Input: part model. Units: mm. Frame: model coordinates. A direction names the side the tool comes from. Round coordinates to 2 decimals unless told otherwise and drop trailing zeros. Order: outer loops, then holes, each group sorted by start corner. A loop starts at its lowest first (then second) coordinate and runs counter-clockwise, first axis right, second up. Notation, with made-up numbers: (50.25, 31.25) -> (59.25, 31.25) arc R31 ccw to (59.25, 60.25) -> close; hole circle Ø3 at (24.5, 38). An arc over 180 degrees is marked (long way). Use a Markdown table: item, result.
from build123d import *

# Parameters (mm, degrees)
F1_R     = 11
F1_R_2   = 5
F1_R_3   = 4.125
F2_DEPTH = 3
F3_START = 2
F3_DEPTH = 6
F4_START = 3
F4_DEPTH = 1.5
F5_SIZE  = 1
F6_R     = 1
F7_R     = 1.99999


# Not quite as in the source:
# - a fillet or chamfer that OpenCascade refuses, or shapes differently, is made with other operations: its cross-section is extruded or revolved along the edge and cut away or added
# - a fillet or chamfer is up to 0.001 mm smaller than in the source, because OpenCascade refuses the exact size


with BuildPart() as f2:
    # F1 (on Top) → F2 (new body)
    with BuildSketch(Plane.XY):
        Circle(F1_R)
        Circle(F1_R_2, mode=Mode.SUBTRACT)
        Circle(F1_R_2)
        Circle(F1_R_3, mode=Mode.SUBTRACT)
    extrude(amount=F2_DEPTH)

    # F1 (on Top) → F3 (join)
    with BuildSketch(Plane.XY.offset(F3_START)):
        Circle(F1_R_3)
    extrude(amount=F3_DEPTH)

    # F1 (on Top) → F4 (join)
    with BuildSketch(Plane.XY.offset(F4_START)):
        Circle(F1_R_2)
        Circle(F1_R_3, mode=Mode.SUBTRACT)
    extrude(amount=F4_DEPTH)

    # F5
    f5_edges = [f2.edges().sort_by_distance(p)[0] for p in [
        (-4.125, 0, 8),
    ]]
    chamfer(f5_edges, length=F5_SIZE)

    # F6
    f6_edges = [f2.edges().sort_by_distance(p)[0] for p in [
        (-11, 0, 0),
    ]]
    fillet(f6_edges, radius=F6_R)

    # F7 (radius 2 in the source; OpenCascade refuses exactly that, so slightly less here)
    f7_edges = [f2.edges().sort_by_distance(p)[0] for p in [
        (-11, 0, 3),
    ]]
    fillet(f7_edges, radius=F7_R)

    # F8: fillet of radius 8 on 1 edges, made by hand

    # F8_s1 → F8_t2 (revolve, cut)
    with BuildSketch(Plane.XZ):
        with BuildLine():
            ThreePointArc((9.4165026221, 0), (6.5880754974, 0.5166852265), (4.125, 2))
            Line((4.125, 2), (4.0191699476, 1.88))
            ThreePointArc((4.0191699476, 1.88), (3.965, 1), (3.965, 0))
            Line((3.965, 0), (4.125, -0.16))
            Line((4.125, -0.16), (9.4165026221, -0.16))
            Line((9.4165026221, -0.16), (9.4165026221, 0))
        make_face()
    revolve(axis=Axis((0, 0, 0), (0, 0, 1)), mode=Mode.SUBTRACT)


solid = f2.part
1) Cut plane C-C on z = 2.5. Return loops of the section in (x, y), and give its area (3 significant figures).
Answer key:
| item | result |
|---|---|
| outline | circle Ø20.65 at (0, 0) |
| area | 335 mm^2 |
2) Contact query for flat-ended pins moving along their axis: P1, Ø9, axis at x = 0, y = -1.5, coming from the -Z side; P2, Ø2, axis at x = 7.5, z = 2.5, coming from the -Y side; P3, Ø1, axis at y = -0.5, z = 6, coming from the -X side (3 decimals). Output: stop coordinate, or through.
Answer key:
| item | result |
|---|---|
| P1 | stops at z = 0.77 |
| P2 | stops at y = -8.45 |
| P3 | stops at x = -4.125 |
3) Draft query along Y for faces 1 (the face through (-2, 4, 4.5)), 2 (the face through (-1.08, -4.88, 3.74)), 3 (the face through (0, 0, 2)). Return one class per face: released by +Y, released by -Y, zero draft, split by the parting line, or undercut.
Answer key:
| item | result |
|---|---|
| face 1 | zero draft |
| face 2 | split by the parting line |
| face 3 | undercut |
4) Cut plane D-D on z = 0.5. Return loops of the section in (x, y).
Answer key:
| item | result |
|---|---|
| outline | circle Ø21.73 at (0, 0); hole circle Ø13.27 at (0, 0) |
5) Set-up query: faces 4 (the face through (4, -4, 3)), 5 (the face through (0, 0, 8)). Return all of +Z, -Z, +X, -X, +Y, -Y with unobstructed straight access to the full face (end or side cutting, diameter ignored); none if empty.
Answer key:
| item | result |
|---|---|
| face 4 | +Z |
| face 5 | +Z, +X, -X, +Y, -Y |
6) Ray query, probe 1 along Y at (x, z) = (3.25, 1.75); probe 2 along Y at (x, z) = (0, 5.75) (3 decimals); probe 3 along Y at (x, z) = (0, 7.5) (3 decimals). Return the intervals inside material, ascending.
Answer key:
| item | result |
|---|---|
| probe 1 | y = -10.36 to -3, 3 to 10.36 |
| probe 2 | y = -4.125 to 4.125 |
| probe 3 | y = -3.625 to 3.625 |
